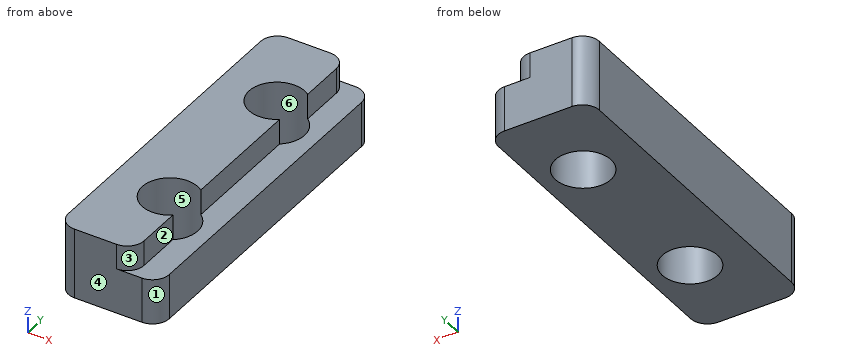
from build123d import *

# Parameters (mm, degrees)
SKETCH_W     = 6
SKETCH_H     = 20
SKETCH_R     = 1.65
PAD_DEPTH    = 2.7
SKETCH001_W  = 4.5
SKETCH001_H  = 20
PAD001_DEPTH = 1.5
SKETCH002_R  = 1.65
POCKET_DEPTH = 4.201
FILLET_R     = 1


with BuildPart() as part:
    # Sketch → Pad (new body)
    with BuildSketch(Plane.XY):
        with Locations((-0.5, -5)):
            Rectangle(SKETCH_W, SKETCH_H)
        Circle(SKETCH_R, mode=Mode.SUBTRACT)
        with Locations((0, -10)):
            Circle(SKETCH_R, mode=Mode.SUBTRACT)
    extrude(amount=PAD_DEPTH)

    # Sketch001 (on Face8 of Pad) → Pad001 (join)
    with BuildSketch(Plane.XY.offset(2.7)):
        with Locations((-1.25, -5)):
            Rectangle(SKETCH001_W, SKETCH001_H)
    extrude(amount=PAD001_DEPTH)

    # Sketch002 → Pocket (cut, through all)
    with BuildSketch(Plane.XY.offset(4.2)):
        Circle(SKETCH002_R)
        with Locations((0, -10)):
            Circle(SKETCH002_R)
    extrude(amount=-POCKET_DEPTH, mode=Mode.SUBTRACT)

    # Fillet
    fillet_edges = [part.edges().sort_by_distance(p)[0] for p in [
        (-3.5, -15, 3.45),
        (-3.5, -15, 1.35),
        (-3.5, 5, 3.45),
        (-3.5, 5, 1.35),
        (2.5, -15, 1.35),
        (1, -15, 3.45),
        (2.5, 5, 1.35),
        (1, 5, 3.45),
    ]]
    fillet(fillet_edges, radius=FILLET_R)


solid = part.part
Geometry check sheet. Reference: the model listing, model coordinates, mm. Face numbers are marked on the shaded views. A direction names the side the tool comes from. Coordinates: 2 decimals unless noted, no trailing zeros. Order: outer loops, then holes, each group sorted by start corner. A loop starts at its lowest first (then second) coordinate and runs counter-clockwise, first axis right, second up. Notation, with made-up numbers: (-6, 10) -> (14, 10) arc R13 ccw to (14, 29) -> close; hole circle Ø7 at (63.5, 69.5). An arc over 180 degrees is marked (long way). Use a Markdown table: item, result. Add a question column.
1. Go/stop test with a flat-tipped pin: pin 1 Ø0.8 at (y, z) = (3, 3.5) entering from +X. Record where the tip stops, or that it passes through.
2. Mould release check, pull along X, two halves, no side actions. Record for the marked faces 3, 4, 5 and 6: pulls with the +X half, pulls with the -X half, needs draft (parallel to the pull), parting line crosses it, or undercut.
3. Material ranges on L1, parallel to Y at x = 0, z = 2.05; L2, parallel to X at y = 0, z = 2.5; L3, parallel to Y at x = -1.45, z = 3.95, recorded low to high.
4. Cross-section at A-A (y = 0). Enter the section's corners in (x, z).
5. Cross-section at D-D (y = -11). Enter the section's corners in (x, z).
6. Set-up check for the marked faces 1 and 2: record each of +Z, -Z, +X, -X, +Y, -Y from which the full face is reachable in a straight line by a thin tool's end or side.
7. Cross-section at B-B (z = 1.55). Enter the section's corners in (x, y), and give its area (3 significant figures).
8. Cross-section at C-C (x = -0.2). Enter the section's corners in (y, z), and give its area (3 significant figures).
Filled sheet:
| question | item | result |
|---|---|---|
| 1 | pin 1 | x = 1 |
| 2 | face 3 | pulls with the +X half |
| 2 | face 4 | needs draft |
| 2 | face 5 | undercut |
| 2 | face 6 | undercut |
| 3 | L1 | -15 to -11.65, -8.35 to -1.65, 1.65 to 5 |
| 3 | L2 | -3.5 to -1.65, 1.65 to 2.5 |
| 3 | L3 | -15 to -10.79, -9.21 to -0.79, 0.79 to 5 |
| 4 | outline | (-3.5, 0) -> (-1.65, 0) -> (-1.65, 4.2) -> (-3.5, 4.2) -> close; (1.65, 0) -> (2.5, 0) -> (2.5, 2.7) -> (1.65, 2.7) -> close |
| 5 | outline | (-3.5, 0) -> (-1.31, 0) -> (-1.31, 4.2) -> (-3.5, 4.2) -> close; (1.31, 0) -> (2.5, 0) -> (2.5, 2.7) -> (1.31, 2.7) -> close |
| 6 | face 1 | +Z, -Z, +X, -Y |
| 6 | face 2 | +Z, +X, +Y, -Y |
| 7 | outline | (-3.5, -14) arc R1 ccw to (-2.5, -15) -> (1.5, -15) arc R1 ccw to (2.5, -14) -> (2.5, 4) arc R1 ccw to (1.5, 5) -> (-2.5, 5) arc R1 ccw to (-3.5, 4) -> close; hole circle Ø3.3 at (0, -10); hole circle Ø3.3 at (0, 0) |
| 7 | area | 102 mm2 |
| 8 | outline | (-15, 0) -> (-11.64, 0) -> (-11.64, 4.2) -> (-15, 4.2) -> close; (-8.36, 0) -> (-1.64, 0) -> (-1.64, 4.2) -> (-8.36, 4.2) -> close; (1.64, 0) -> (5, 0) -> (5, 4.2) -> (1.64, 4.2) -> close |
| 8 | area | 56.5 mm2 |
